Verification items for the finished model (mm, model axes). Face numbers are marked on the shaded views. Give positions to 0.01 mm unless a question says otherwise; leave off trailing zeros. Loops run counter-clockwise (first coordinate to the right, second up) from the corner with the lowest first, then second, coordinate; pieces in that order, holes last. Notation, with made-up numbers: (4, 82) - (49, 82) arc R33 cw to (49, 117) - close; hole circle Ø7 at (75.5, -37). An arc over 180 degrees is marked (long way). Answer in a Markdown table with one row per item.
```python
from build123d import *

# Parameters (mm, degrees)
SKETCH1_R           = 4.7625
SKETCH1_W           = 38.80104
SKETCH1_H           = 38.80104
SKETCH1_R_2         = 3.175
BOSS_EXTRUDE1_DEPTH = 6.35
FILLET1_R           = 6.35


with BuildPart() as part:
    # Sketch1 → Boss-Extrude1 (new body)
    with BuildSketch(Plane.XY):
        Polygon((19.40052, 19.40052), (-19.40052, 19.40052), (-19.40052, 44.4390625), (-19.40052, 83.2401025), (19.40052, 83.2401025), (19.40052, 44.4390625), align=None)
        with Locations((0, 63.8395825)):
            Circle(SKETCH1_R, mode=Mode.SUBTRACT)
        Rectangle(SKETCH1_W, SKETCH1_H)
        with Locations((13.05052, -13.05052)):
            Circle(SKETCH1_R_2, mode=Mode.SUBTRACT)
        with Locations((-13.05052, -13.05052)):
            Circle(SKETCH1_R_2, mode=Mode.SUBTRACT)
        with Locations((-13.05052, 13.05052)):
            Circle(SKETCH1_R_2, mode=Mode.SUBTRACT)
        with Locations((13.05052, 13.05052)):
            Circle(SKETCH1_R_2, mode=Mode.SUBTRACT)
    extrude(amount=BOSS_EXTRUDE1_DEPTH)

    # Fillet1
    fillet1_edges = [part.edges().sort_by_distance(p)[0] for p in [
        (-19.40052, 83.2401025, 3.175),
        (19.40052, 83.2401025, 3.175),
    ]]
    fillet(fillet1_edges, radius=FILLET1_R)


solid = part.part
```
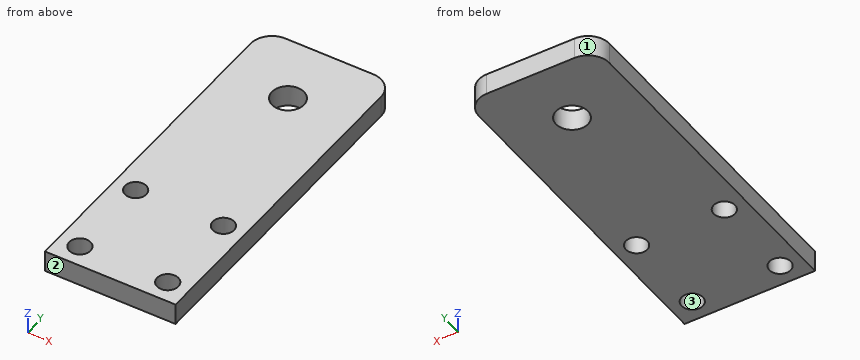
Q1. Draft check along X on the marked faces 1, 2 and 3. Enter one of: +X half, -X half, draft (parallel to the pull), parting line (faces both ways), or undercut.
Completed:
| item | result |
|---|---|
| face 1 | -X half |
| face 2 | draft |
| face 3 | undercut |
Q2. Sectioned sample at B-B (z = 4). Give the number of separate pieces and of enclosed holes in the cut face, and give its area (3 significant figures).
Completed:
| item | result |
|---|---|
| separate pieces | 1 |
| enclosed holes | 5 |
| area | 3,770 mm^2 |
Q3. Sectioned sample at A-A (x = 0). Record the cut outline in (y, z).
Completed:
| item | result |
|---|---|
| outline | (-19.4, 0) - (59.08, 0) - (59.08, 6.35) - (-19.4, 6.35) - close; (68.6, 0) - (83.24, 0) - (83.24, 6.35) - (68.6, 6.35) - close |
Q4. Thickness scan on line 1 (X direction, y = -14.5, z = 6.25); line 2 (Y direction, x = -11, z = 5.5); line 3 (Y direction, x = -14, z = 3.75). Record the ranges inside material, lowest first.
Completed:
| item | result |
|---|---|
| line 1 | -19.4 to -15.88, -10.23 to 10.23, 15.88 to 19.4 |
| line 2 | -19.4 to -15.47, -10.63 to 10.63, 15.47 to 83.24 |
| line 3 | -19.4 to -16.08, -10.02 to 10.02, 16.08 to 83.17 |
